Part model, mm, in its own coordinate system. Give positions to 0.01 mm unless a question says otherwise; leave off trailing zeros. Write each loop counter-clockwise with the first axis right and the second up, starting at its lowest first coordinate (ties: lowest second). Pieces come first, ordered by that corner, then holes.
Autodesk Inventor part; units mm, degrees
ref_plane "YZ Plane" through (0, 0, 0) normal (1, 0, 0) x (0, 1, 0)
ref_plane "XZ Plane" through (0, 0, 0) normal (0, 1, 0) x (-1, 0, 0)
ref_plane "XY Plane" through (0, 0, 0) normal (0, 0, 1) x (1, 0, 0)
sketch "Sketch1" plane through (0, 0, 0) normal (0, 0, 1) x (1, 0, 0)
  arc A0 (-179.9924, 22) -> (-183.6588, 16.912) centre (-179.5223, 17.7962) ccw
  arc A1 (-183.6588, -17.77) -> (-179.4288, -22) centre (-179.4288, -17.77) ccw
  arc A2 (-48.2588, 16.912) -> (-52.4305, 22) centre (-52.4009, 17.7701) ccw
  arc A3 (-52.9925, -22) -> (-48.2588, -17.77) centre (-52.4887, -17.8001) ccw
  line L0 (-52.4305, 22) -> (-179.9924, 22)
  line L1 (-52.9925, -22) -> (-179.4288, -22)
  line L2 (-48.2588, -17.77) -> (-48.2588, 16.912)
  line L3 (-183.6588, -17.77) -> (-183.6588, 16.912)
  line L4 (-286.5288, -25.829) -> (-208.4238, -25.829)
  line L5 (-286.5288, 24.971) -> (-208.4238, 24.971)
  line L6 (-205.2488, 21.796) -> (-205.2488, -22.654)
  arc A4 (-205.2488, 21.796) -> (-208.4238, 24.971) centre (-208.4238, 21.796) ccw
  arc A5 (-208.4238, -25.829) -> (-205.2488, -22.654) centre (-208.4238, -22.654) ccw
  arc A6 (44.1612, -17.77) -> (48.3912, -22) centre (48.3912, -17.77) ccw
  arc A7 (47.8276, 22) -> (44.1612, 16.912) centre (48.2978, 17.7962) ccw
  line L7 (44.1612, -17.77) -> (44.1612, 16.912)
  line L8 (204.3262, 25.4) -> (282.4312, 25.4)
  line L9 (204.3262, -25.4) -> (282.4312, -25.4)
  line L10 (174.8276, -22) -> (48.3912, -22)
  line L11 (175.3896, 22) -> (47.8276, 22)
  arc A8 (179.5612, 16.912) -> (175.3896, 22) centre (175.4192, 17.7701) ccw
  line L12 (179.5612, -17.77) -> (179.5612, 16.912)
  arc A9 (174.8276, -22) -> (179.5612, -17.77) centre (175.3313, -17.8001) ccw
  arc A10 (201.1512, -22.225) -> (204.3262, -25.4) centre (204.3262, -22.225) ccw
  arc A11 (204.3262, 25.4) -> (201.1512, 22.225) centre (204.3262, 22.225) ccw
  line L13 (201.1512, 22.225) -> (201.1512, -22.225)
  line L14 (-286.5288, 38.1) -> (282.4312, 38.1)
  line L15 (-286.5288, -38.1) -> (282.4312, -38.1)
  line L16 (282.4312, 38.1) -> (282.4312, 25.4)
  line L17 (282.4312, -25.4) -> (282.4312, -38.1)
  line L18 (-286.5288, 38.1) -> (-286.5288, 24.971)
  line L19 (-286.5288, -25.829) -> (-286.5288, -38.1)
  dimension "d0" = 135.4
  dimension "d1" = 44
  dimension "d8" = 78.105
  dimension "d13" = 50.8
  dimension "d14" = 44.45
  dimension "d15" = 21.59
  dimension "d18" = 135.4
  dimension "d19" = 44
  dimension "d20" = 78.105
  dimension "d21" = 50.8
  dimension "d26" = 568.96
  dimension "d33" = 21.59
extrude "Extrusion2" add sketch "Sketch1" along normal blind 9.525
properties part number "top" material "Aluminum 6061"
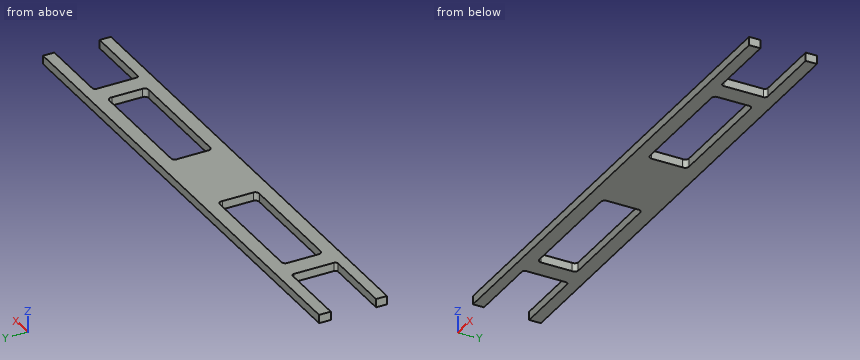
1) Drill centre lines: L1, parallel to X at y = 15, z = 2.25; L2, parallel to Y at x = -148, z = 4; L3, parallel to Y at x = 210.5, z = 3. Where is each one in solid material? Low to high.
Check result:
L1: x = -205.25 to -183.66, -48.26 to 44.16, 179.56 to 201.15
L2: y = -38.1 to -22, 22 to 38.1
L3: y = -38.1 to -25.4, 25.4 to 38.1
2) Saw through at C-C (x = -241). Write the cut outline in (y, z) (3 decimals), and give its area (3 significant figures).
Check result:
outline: (-38.1, 0) - (-25.829, 0) - (-25.829, 9.525) - (-38.1, 9.525) - close; (24.971, 0) - (38.1, 0) - (38.1, 9.525) - (24.971, 9.525) - close
area: 242 mm2
3) Saw through at B-B (z = 8). State how many separate pieces and enclosed holes the cut face has, and give its area (3 significant figures).
Check result:
separate pieces: 1
enclosed holes: 2
area: 23,200 mm2
4) Flat gauge pins, fed straight in: P1, Ø1.5, axis at y = -5.5, z = 2.5, coming from the -X side; P2, Ø4, axis at y = 5, z = 3, coming from the +X side. Where does each tip first touch, or does it go through?
Check result:
P1: stops at x = -205.25
P2: stops at x = 201.15
5) Saw through at A-A (y = -1). Write the cut outline in (x, z) (3 decimals).
Check result:
outline: (-205.249, 0) - (-183.659, 0) - (-183.659, 9.525) - (-205.249, 9.525) - close; (-48.259, 0) - (44.161, 0) - (44.161, 9.525) - (-48.259, 9.525) - close; (179.561, 0) - (201.151, 0) - (201.151, 9.525) - (179.561, 9.525) - close
6) Saw through at D-D (x = 95.5). Write the cut outline in (y, z) (3 decimals).
Check result:
outline: (-38.1, 0) - (-22, 0) - (-22, 9.525) - (-38.1, 9.525) - close; (22, 0) - (38.1, 0) - (38.1, 9.525) - (22, 9.525) - close
